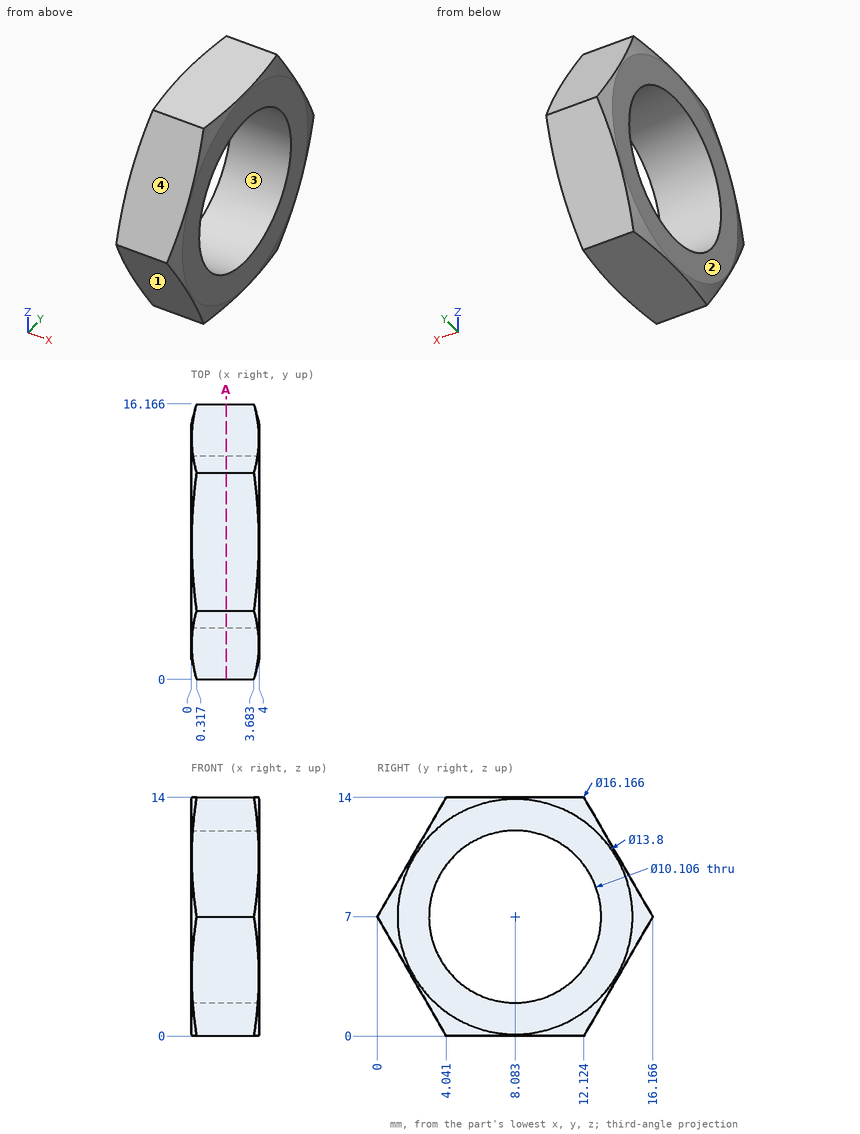
Design review of the part shown in the three views and the two pictorial views. Dimensions are in mm from the part's minimum x, y and z. Round coordinates to 2 decimals unless told otherwise and drop trailing zeros. Write each loop counter-clockwise with the first axis right and the second up, starting at its lowest first coordinate (ties: lowest second). Pieces come first, ordered by that corner, then holes.
Item 1: Consider section A-A on x = 2.05. Give the boundary of the cut face in (y, z) (1 decimal).
Item 2: For pin 1 Ø3 at (y, z) = (5, 6.5) entering from +X, flat-tipped, find the tip position at first contact; note if it passes through.
Item 3: Draft analysis for pull direction Z (two halves, no side actions). For the marked faces 1, 2, 3 and 4, state which applies: released by +Z, released by -Z, zero draft, split by the parting line, or undercut.
Item 4: Wall thickness on L1, parallel to Z at x = 3.85, y = 8.25; L2, parallel to Y at x = 0.7, z = 9.75 (1 decimal); L3, parallel to Z at x = 3.4, y = 9.5: over which ranges is each line inside the solid? List them lowest first.
Check values:
1. outline: (0, 7) - (4, 0) - (12.1, 0) - (16.2, 7) - (12.1, 14) - (4, 14) - close; hole circle Ø10.1 at (8.1, 7)
2. pin 1: passes through
3. face 1: released by -Z
3. face 2: zero draft
3. face 3: undercut
3. face 4: released by +Z
4. L1: z = 0 to 1.95, 12.05 to 14
4. L2: y = 1.6 to 3.8, 12.3 to 14.6
4. L3: z = 0 to 2.15, 11.85 to 14
